Model file for the job. Use its own axes, mm. A direction names the side the tool comes from. Coordinates: 2 decimals unless noted, no trailing zeros. Loops run counter-clockwise (first coordinate to the right, second up) from the corner with the lowest first, then second, coordinate; pieces in that order, holes last. Notation, with made-up numbers: (44, 63.25) -> (80, 63.25) arc R23 cw to (80, 88.25) -> close; hole circle Ø1 at (19, 88.5). An arc over 180 degrees is marked (long way). Use one line per item in the form item = value.
```python
from build123d import *

# Parameters (mm, degrees)
CROQUIS1_W              = 40
CROQUIS1_H              = 70
SALIENTE_EXTRUIR1_DEPTH = 5
CROQUIS3_W              = 48
CROQUIS3_H              = 78
SALIENTE_EXTRUIR3_DEPTH = 3
CROQUIS5_W              = 35
CROQUIS5_H              = 70
CORTAR_EXTRUIR1_DEPTH   = 5


with BuildPart() as part:
    # Croquis1 → Saliente-Extruir1 (new body)
    with BuildSketch(Plane(origin=(0, 0, 0), x_dir=(1, 0, 0), z_dir=(0, 1, 0))):
        with Locations((-20, -35)):
            Rectangle(CROQUIS1_W, CROQUIS1_H)
    extrude(amount=SALIENTE_EXTRUIR1_DEPTH)

    # Croquis3 → Saliente-Extruir3 (add)
    with BuildSketch(Plane(origin=(0, 5, 0), x_dir=(1, 0, 0), z_dir=(0, 1, 0))):
        with Locations((-20, -35)):
            Rectangle(CROQUIS3_W, CROQUIS3_H)
    extrude(amount=SALIENTE_EXTRUIR3_DEPTH)

    # Croquis5 → Cortar-Extruir1 (cut)
    with BuildSketch(Plane.XZ):
        with Locations((-20, 35)):
            Rectangle(CROQUIS5_W, CROQUIS5_H)
    extrude(amount=-CORTAR_EXTRUIR1_DEPTH, mode=Mode.SUBTRACT)


solid = part.part
```
Q1. Band-saw the part on B-B, the plane z = 5.5. Write the cut outline in (x, y), and give its area (3 significant figures).
Result:
outline = (-44, 5) -> (-40, 5) -> (-40, 0) -> (-37.5, 0) -> (-37.5, 5) -> (-2.5, 5) -> (-2.5, 0) -> (0, 0) -> (0, 5) -> (4, 5) -> (4, 8) -> (-44, 8) -> close
area = 169 mm2
Q2. Pin check, flat tips, straight feed: pin 1 Ø1.5 at (y, z) = (2.5, 31) entering from +X; pin 2 Ø2 at (x, y) = (-1.5, 3.5) entering from -Z; pin 3 Ø2.5 at (y, z) = (2, 52.5) entering from -X. Stop position of each tip, or through.
Result:
pin_1 = 0
pin_2 = 0
pin_3 = -40
Q3. Band-saw the part on C-C, the plane x = -1. Write the cut outline in (y, z).
Result:
outline = (0, 0) -> (5, 0) -> (5, -4) -> (8, -4) -> (8, 74) -> (5, 74) -> (5, 70) -> (0, 70) -> close
Q4. Band-saw the part on A-A, the plane y = 3. Write the cut outline in (x, z).
Result:
outline = (-40, 0) -> (-37.5, 0) -> (-37.5, 70) -> (-40, 70) -> close; (-2.5, 0) -> (0, 0) -> (0, 70) -> (-2.5, 70) -> close
Q5. Band-saw the part on D-D, the plane x = -10. Write the cut outline in (y, z).
Result:
outline = (5, -4) -> (8, -4) -> (8, 74) -> (5, 74) -> close
Q6. Which spindle directions (+Z, -Z, +X, -X, +Y, -Y) get a long thin tool onto all of the face, cutting with end or side? Do faces 1 (the face through (-39, 2, 70)), 2 (the face through (-1, 2, 0)), 3 (the face through (0, 2, 35)). Say none if no direction does.
Result:
face_1 = +Z, +X, -X, -Y
face_2 = -Z, +X, -X, -Y
face_3 = +Z, -Z, +X, -Y
Q7. Mould opens along X. For faces 4 (the face through (-2.5, 2, 35)), 5 (the face through (-39, 2, 0)), 6 (the face through (4, 6, 36)) say: released by +X, released by -X, zero draft, split by the parting line, or undercut.
Result:
face_4 = undercut
face_5 = zero draft
face_6 = released by +X
Q8. Wall check: line 1 along X through (y, z) = (2.25, 15); line 2 along Y through (x, z) = (-17, 3); line 3 along Z through (x, y) = (-2, 1.75). Give the ranges that are in metal, low to high.
Result:
line_1 = -40 to -37.5, -2.5 to 0
line_2 = 5 to 8
line_3 = 0 to 70
